Read the model definition and answer for the solid it produces. Units are mm, in the model's axes. A direction names the side the tool comes from. Round coordinates to 2 decimals unless told otherwise and drop trailing zeros. Order: outer loops, then holes, each group sorted by start corner. A loop starts at its lowest first (then second) coordinate and runs counter-clockwise, first axis right, second up. Notation, with made-up numbers: (11, -37.75) - (53, -37.75) arc R34 cw to (53, -4.75) - close; hole circle Ø6 at (-17, 29). An arc over 180 degrees is marked (long way). Answer as a JSON object with one key per item and string values. Group by question number.
Q1. The mould has two halves that part along Z. Classify faces 1 (the flat face through (2, -6, 5)), 2 (the flat face through (2, -3, 0)), 3 (the flat face through (3, -4.25, 8)): pulls with the +Z half, pulls with the -Z half, needs draft (parallel to the pull), parting line crosses it, or undercut.
Q2. A tool of negligible diameter and unlimited length cuts with its end or side. For faces 4 (the flat face through (2, 0, 5)), 5 (the cylindrical face through (2.82, -5.14, 7.2)), 6 (the flat face through (3, -3.25, 2)), from which of +Z, -Z, +X, -X, +Y, -Y can it reach the whole face along a straight path? Write none if from no direction.
Q3. A cutting plane is placed at C-C on y = -2.7. Determine the outline of the cut face in (x, z).
Q4. A cutting plane is placed at D-D on x = 2.5. Determine the outline of the cut face in (y, z), and give its area (3 significant figures).
Q5. A cutting plane is placed at B-B on z = 6. Determine the outline of the cut face in (x, y), and give its area (3 significant figures).
Q6. A cutting plane is placed at A-A on y = -3.5. Determine the outline of the cut face in (x, z), and give its area (3 significant figures).
Q7. Consider line 1 (Z direction, x = 3.8, y = -3.5); line 2 (X direction, y = -1.3, z = 1.8); line 3 (Y direction, x = 2.45, z = 8.75). Determine where each line is inside the solid, lowest interval first.
Q8. Given pin 1 Ø1.7 at (x, z) = (2.5, 8.2) entering from -Y; pin 2 Ø1.9 at (x, z) = (2.5, 1.8) entering from +Y, each flat-ended and moving along its own axis, determine where each tip first touches the part or whether it passes through.
```python
from build123d import *

# Parameters (mm, degrees)
SKETCH1_W           = 5
SKETCH1_H           = 6
BOSS_EXTRUDE1_DEPTH = 10
CUT_EXTRUDE1_REACH  = 14.689
SKETCH2_R           = 1.5
SKETCH3_R           = 1.05
CUT_EXTRUDE2_DEPTH  = 3.25
SKETCH4_R           = 1.05
CUT_EXTRUDE3_DEPTH  = 1.75


with BuildPart() as part:
    # Sketch1 → Boss-Extrude1 (new body)
    with BuildSketch(Plane.XY):
        with Locations((2.5, -3)):
            Rectangle(SKETCH1_W, SKETCH1_H)
    extrude(amount=BOSS_EXTRUDE1_DEPTH)

    # Sketch2 → Cut-Extrude1 (cut, up to next)
    with BuildSketch(Plane(origin=(5, 0, 0), x_dir=(0, 0, -1), z_dir=(1, 0, 0)), mode=Mode.PRIVATE) as cut_extrude1_sk1:
        with Locations(Location((-5, -3.5, 0), (0, 0, 90))):
            Circle(SKETCH2_R)
    cut_extrude1_tool1 = extrude(cut_extrude1_sk1.sketch, amount=-CUT_EXTRUDE1_REACH, mode=Mode.PRIVATE) & part.part
    add(cut_extrude1_tool1.solids().sort_by_distance((5, -3.5, 5))[0], mode=Mode.SUBTRACT)

    # Sketch3 → Cut-Extrude2 (cut)
    with BuildSketch(Plane(origin=(0, 0, 0), x_dir=(1, 0, 0), z_dir=(0, 1, 0))):
        with Locations(Location((2.5, -1.8, 0), (0, 0, 270))):
            Circle(SKETCH3_R)
    extrude(amount=-CUT_EXTRUDE2_DEPTH, mode=Mode.SUBTRACT)

    # Sketch4 → Cut-Extrude3 (cut)
    with BuildSketch(Plane.XZ.offset(6)):
        with Locations(Location((2.5, 8.2, 0), (0, 0, 270))):
            Circle(SKETCH4_R)
    extrude(amount=-CUT_EXTRUDE3_DEPTH, mode=Mode.SUBTRACT)


solid = part.part
```
Result set:
{
 "1": {"face 1": "needs draft", "face 2": "pulls with the -Z half", "face 3": "undercut"},
 "2": {"face 4": "+Z, -Z, +X, -X, +Y", "face 5": "-Y", "face 6": "+Y"},
 "3": {"outline": "(0, 0) - (5, 0) - (5, 3.73) - (0, 3.73) - close; (0, 6.27) - (5, 6.27) - (5, 10) - (0, 10) - close; hole circle Ø2.1 at (2.5, 1.8)"},
 "4": {"outline": "(-6, 0) - (0, 0) - (0, 0.75) - (-3.25, 0.75) - (-3.25, 2.85) - (0, 2.85) - (0, 10) - (-6, 10) - (-6, 9.25) - (-4.25, 9.25) - (-4.25, 7.15) - (-6, 7.15) - close; hole circle Ø3 at (-3.5, 5)", "area": "42.4 mm²"},
 "5": {"outline": "(0, -6) - (5, -6) - (5, -4.62) - (0, -4.62) - close; (0, -2.38) - (5, -2.38) - (5, 0) - (0, 0) - close", "area": "18.8 mm²"},
 "6": {"outline": "(0, 0) - (5, 0) - (5, 3.5) - (0, 3.5) - close; (0, 6.5) - (5, 6.5) - (5, 10) - (0, 10) - close", "area": "35.0 mm²"},
 "7": {"line 1": "z = 0 to 3.5, 6.5 to 10", "line 2": "x = 0 to 1.45, 3.55 to 5", "line 3": "y = -4.25 to 0"},
 "8": {"pin 1": "stops at y = -4.25", "pin 2": "stops at y = -3.25"}
}
